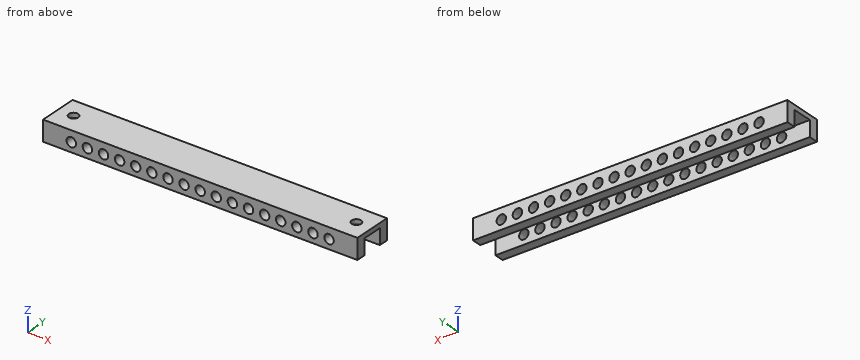
```python
from build123d import *

# Parameters (mm, degrees)
SKETCH1_W               = 100
SKETCH1_H               = 12.5
BOSS_EXTRUDE1_DEPTH     = 1.5
SKETCH2_W               = 100
SKETCH2_H               = 3
BOSS_EXTRUDE2_DEPTH     = 5
CUT_EXTRUDE1_DEPTH      = 52.780787943
CUT_EXTRUDE1_DEPTH_BACK = 52.780787943
SKETCH3_R               = 1.5
SKETCH4_R               = 1.5
CUT_EXTRUDE2_DEPTH      = 51.636572751


with BuildPart() as part:
    # Sketch1 → Boss-Extrude1 (new body)
    with BuildSketch(Plane.XY):
        Rectangle(SKETCH1_W, SKETCH1_H)
    extrude(amount=BOSS_EXTRUDE1_DEPTH)

    # Sketch2 → Boss-Extrude2 (add)
    with BuildSketch(Plane(origin=(0, 0, 0), x_dir=(-1, 0, 0), z_dir=(0, 0, -1))):
        with Locations((0, 4.75)):
            Rectangle(SKETCH2_W, SKETCH2_H)
        with Locations((0, -4.75)):
            Rectangle(SKETCH2_W, SKETCH2_H)
    extrude(amount=BOSS_EXTRUDE2_DEPTH)

    # Sketch3 → Cut-Extrude1 (cut, two sides: drawn at the far end of the back side and taken through both)
    with BuildSketch(Plane.XZ.offset(6.25).offset(-CUT_EXTRUDE1_DEPTH_BACK)):
        with Locations((41, -2)):
            Circle(SKETCH3_R)
        with Locations((35.875, -2)):
            Circle(SKETCH3_R)
        with Locations((30.75, -2)):
            Circle(SKETCH3_R)
        with Locations((25.625, -2)):
            Circle(SKETCH3_R)
        with Locations((20.5, -2)):
            Circle(SKETCH3_R)
        with Locations((15.375, -2)):
            Circle(SKETCH3_R)
        with Locations((10.25, -2)):
            Circle(SKETCH3_R)
        with Locations((5.125, -2)):
            Circle(SKETCH3_R)
        with Locations((0, -2)):
            Circle(SKETCH3_R)
        with Locations((-5.125, -2)):
            Circle(SKETCH3_R)
        with Locations((-10.25, -2)):
            Circle(SKETCH3_R)
        with Locations((-15.375, -2)):
            Circle(SKETCH3_R)
        with Locations((-20.5, -2)):
            Circle(SKETCH3_R)
        with Locations((-25.625, -2)):
            Circle(SKETCH3_R)
        with Locations((-30.75, -2)):
            Circle(SKETCH3_R)
        with Locations((-35.875, -2)):
            Circle(SKETCH3_R)
        with Locations((-41, -2)):
            Circle(SKETCH3_R)
    extrude(amount=CUT_EXTRUDE1_DEPTH + CUT_EXTRUDE1_DEPTH_BACK, mode=Mode.SUBTRACT)

    # Sketch4 → Cut-Extrude2 (cut, through all)
    with BuildSketch(Plane(origin=(0, 0, 0), x_dir=(-1, 0, 0), z_dir=(0, 0, -1))):
        with Locations((-45, 0)):
            Circle(SKETCH4_R)
        with Locations(Location((45, 0, 0), (0, 0, 180))):
            Circle(SKETCH4_R)
    extrude(amount=-CUT_EXTRUDE2_DEPTH, mode=Mode.SUBTRACT)


solid = part.part
```
Part model, mm, in its own coordinate system. Round coordinates to 2 decimals unless told otherwise and drop trailing zeros. Loops run counter-clockwise (first coordinate to the right, second up) from the corner with the lowest first, then second, coordinate; pieces in that order, holes last.
Item 1: Cut at B-B, the plane y = -5.25. State how many separate pieces and enclosed holes the cut face has, then the cut area to 3 significant figures.
Item 2: Drill centre lines: line 1 (Y direction, x = -13.5, z = -3.25); line 2 (Z direction, x = -41, y = -5.2); line 3 (Y direction, x = -45, z = 1.15). Where is each one in solid material? Low to high.
Item 3: Cut at D-D, the plane x = -10. Give the cut face in (y, z), then the cut area to 3 significant figures.
Item 4: Cut at C-C, the plane y = 0. Give the cut face in (x, z), then the cut area to 3 significant figures.
Item 5: Drop a flat-ended pin along its axis: P1, Ø1, axis at y = -2, z = -1, coming from the -X side. Give the stop position or say it passes through.
Item 6: Cut at A-A, the plane x = 45. Give the cut face in (y, z), then the cut area to 4 significant figures.
A:
1. separate pieces: 1
1. enclosed holes: 17
1. area: 530 mm2
2. line 1: y = -6.25 to -3.25, 3.25 to 6.25
2. line 2: z = -5 to -3.5, -0.5 to 1.5
2. line 3: y = -6.25 to -1.5, 1.5 to 6.25
3. outline: (-6.25, -5) - (-3.25, -5) - (-3.25, -3.48) - (-6.25, -3.48) - close; (-6.25, -0.52) - (-3.25, -0.52) - (-3.25, 0) - (3.25, 0) - (3.25, -0.52) - (6.25, -0.52) - (6.25, 1.5) - (-6.25, 1.5) - close; (3.25, -5) - (6.25, -5) - (6.25, -3.48) - (3.25, -3.48) - close
3. area: 31.0 mm2
4. outline: (-50, 0) - (-46.5, 0) - (-46.5, 1.5) - (-50, 1.5) - close; (-43.5, 0) - (43.5, 0) - (43.5, 1.5) - (-43.5, 1.5) - close; (46.5, 0) - (50, 0) - (50, 1.5) - (46.5, 1.5) - close
4. area: 141 mm2
5. P1: passes through
6. outline: (-6.25, -5) - (-3.25, -5) - (-3.25, 0) - (-1.5, 0) - (-1.5, 1.5) - (-6.25, 1.5) - close; (1.5, 0) - (3.25, 0) - (3.25, -5) - (6.25, -5) - (6.25, 1.5) - (1.5, 1.5) - close
6. area: 44.25 mm2
